from build123d import *

# Parameters (mm, degrees)
SKETCH021_W  = 50.8
SKETCH021_H  = 93.98
SKETCH021_R  = 1.9
PAD018_DEPTH = 1.5
SKETCH022_W  = 50.8
SKETCH022_H  = 55.6
PAD019_DEPTH = 19
SKETCH023_W  = 50.8
SKETCH023_H  = 15
PAD020_DEPTH = 10


with BuildPart() as part:
    # Sketch021 → Pad018 (new body)
    with BuildSketch(Plane.XZ):
        with Locations((0, 85.19)):
            Rectangle(SKETCH021_W, SKETCH021_H)
        with Locations((-22.225, 129.005)):
            Circle(SKETCH021_R, mode=Mode.SUBTRACT)
        with Locations((22.225, 129.005)):
            Circle(SKETCH021_R, mode=Mode.SUBTRACT)
        with Locations((22.225, 41.375)):
            Circle(SKETCH021_R, mode=Mode.SUBTRACT)
        with Locations((-22.225, 41.375)):
            Circle(SKETCH021_R, mode=Mode.SUBTRACT)
    extrude(amount=PAD018_DEPTH)

    # Sketch022 (on Face10 of Pad018) → Pad019 (join)
    with BuildSketch(Plane.XZ.offset(1.5)):
        with Locations((0, 78.7)):
            Rectangle(SKETCH022_W, SKETCH022_H)
    extrude(amount=PAD019_DEPTH)

    # Sketch023 (on Face4 of Pad019) → Pad020 (join)
    with BuildSketch(Plane(origin=(0, 0, 0), x_dir=(1, 0, 0), z_dir=(0, 1, 0))):
        with Locations((0, -119.38)):
            Rectangle(SKETCH023_W, SKETCH023_H)
    extrude(amount=PAD020_DEPTH)


with BuildPart() as part_1:
    # Body010 placement: moved
    add(part.part.moved(Location((0, 17.7, 0))))


solid = part_1.part
Work out the finished part from the listing and answer in its coordinate system (mm). A direction names the side the tool comes from. Give positions to 0.01 mm unless a question says otherwise; leave off trailing zeros. Write each loop counter-clockwise with the first axis right and the second up, starting at its lowest first coordinate (ties: lowest second). Pieces come first, ordered by that corner, then holes. Notation, with made-up numbers: (71, 78.25) - (128, 78.25) arc R24 ccw to (128, 92.25) - close; hole circle Ø3 at (85, -28). An arc over 180 degrees is marked (long way). One line per item, written item: value. Start each with the question number.
1. Find section C-C (z = 118). Write down the section's boundary in (x, y), then the cut area to 3 significant figures.
2. For faces 1 (the flat face through (0, 17.7, 76)), 2 (the flat face through (0, 17.7, 130)), 3 (the flat face through (0, 16.2, 120)), determine the directions among +Z, -Z, +X, -X, +Y, -Y from which every point of the face is accessible in a straight line to the end or side of a thin tool.
3. For a pull along X with two mould halves and no side action, classify faces 4 (the cylindrical face through (21.98, 16.96, 130.89)), 5 (the flat face through (25.4, 9, 85)), 6 (the flat face through (0, 7, 50.9)) as +X half, -X half, draft (parallel to the pull), parting line (faces both ways), or undercut.
4. Find section A-A (x = 12.5). Write down the section's boundary in (y, z), then the cut area to 3 significant figures.
5. Find section B-B (y = 22). Write down the section's boundary in (x, z).
6. Consider probe 1 along Z at (x, y) = (13, 9.5); probe 2 along Y at (x, z) = (-14.5, 70.5); probe 3 along Y at (x, z) = (19.5, 114). Determine where each line is inside the solid, lowest interval first.
7. Given pin 1 (15 mm diameter, centred on x = -11, y = 8, fed in from +Z); pin 2 (6.5 mm diameter, centred on x = -9, z = 41.5, fed in from -Y); pin 3 (9.5 mm diameter, centred on x = 8, y = 5, fed in from -Z); pin 4 (3 mm diameter, centred on x = -22.225, z = 129.005, fed in from -Y), each flat-ended and moving along its own axis, determine where each tip first touches the part or whether it passes through.
Geometry results:
1. outline: (-25.4, 16.2) - (25.4, 16.2) - (25.4, 27.7) - (-25.4, 27.7) - close
1. area: 584 mm2
2. face 1: -Z, +X, -X, +Y
2. face 2: +Z, +X, -X, +Y
2. face 3: +Z, +X, -X, -Y
3. face 4: undercut
3. face 5: +X half
3. face 6: draft
4. outline: (-2.8, 50.9) - (16.2, 50.9) - (16.2, 38.2) - (17.7, 38.2) - (17.7, 111.88) - (27.7, 111.88) - (27.7, 126.88) - (17.7, 126.88) - (17.7, 132.18) - (16.2, 132.18) - (16.2, 106.5) - (-2.8, 106.5) - close
4. area: 1,350 mm2
5. outline: (-25.4, 111.88) - (25.4, 111.88) - (25.4, 126.88) - (-25.4, 126.88) - close
6. probe 1: 50.9 to 106.5
6. probe 2: -2.8 to 17.7
6. probe 3: 16.2 to 27.7
7. pin 1: z = 106.5
7. pin 2: y = 16.2
7. pin 3: z = 50.9
7. pin 4: through
